Geometry check sheet. Reference: the model listing, model coordinates, mm. A direction names the side the tool comes from. Coordinates: 2 decimals unless noted, no trailing zeros. Loops run counter-clockwise (first coordinate to the right, second up) from the corner with the lowest first, then second, coordinate; pieces in that order, holes last.
from build123d import *

# Parameters (mm, degrees)
F0_W     = 65
F0_H     = 80
F1_DEPTH = 12
F2_T     = 2
F3_W     = 67
F3_H     = 14
F4_DEPTH = 3
F5_W     = 33
F5_H     = 7
F5_W_2   = 39
F5_H_2   = 33
F6_DEPTH = 2


with BuildPart() as f1:
    # F0 (on Front) → F1 (new body)
    with BuildSketch(Plane.XZ):
        with Locations((32.5, 40)):
            Rectangle(F0_W, F0_H)
    extrude(amount=-F1_DEPTH)

    # F2
    f2_openings = [f1.faces().sort_by_distance(p)[0] for p in [
        (32.5, 6, 80),
    ]]
    offset(amount=F2_T, openings=f2_openings, kind=Kind.INTERSECTION)

    # F3 (on face) → F4 (cut)
    with BuildSketch(Plane.XY.offset(80)):
        with Locations((32.5, 6)):
            Rectangle(F3_W, F3_H)
    extrude(amount=-F4_DEPTH, mode=Mode.SUBTRACT)

    # F5 (on face) → F6 (cut, through all)
    with BuildSketch(Plane.XZ.offset(2)):
        with Locations((32.5, 12.5)):
            Rectangle(F5_W, F5_H)
        with Locations((32.5, 56.5)):
            Rectangle(F5_W_2, F5_H_2)
    extrude(amount=-F6_DEPTH, mode=Mode.SUBTRACT)


solid = f1.part
1) Section check A-A on x = 30. Record the cut outline in (y, z).
Data:
outline: (-2, -2) - (14, -2) - (14, 80) - (13, 80) - (13, 77) - (12, 77) - (12, 0) - (0, 0) - (0, 9) - (-2, 9) - close; (-2, 16) - (0, 16) - (0, 40) - (-2, 40) - close; (-2, 73) - (0, 73) - (0, 77) - (-1, 77) - (-1, 80) - (-2, 80) - close
2) Mould release check, pull along X, two halves, no side actions. Record for faces 1 (the flat face through (66, 6, 79)), 2 (the flat face through (32, -2, 39.6)), 3 (the flat face through (-2, 6, 38)): +X half, -X half, draft (parallel to the pull), parting line (faces both ways), or undercut.
Data:
face 1: undercut
face 2: draft
face 3: -X half
3) Section check C-C on y = 10. Record the cut outline in (x, z).
Data:
outline: (-2, -2) - (67, -2) - (67, 80) - (66, 80) - (66, 77) - (65, 77) - (65, 0) - (0, 0) - (0, 77) - (-1, 77) - (-1, 80) - (-2, 80) - close
4) Material ranges on probe 1 along Y at (x, z) = (36, 22.5); probe 2 along X at (y, z) = (2.5, 39); probe 3 along Z at (x, y) = (33.5, 6), recorded low to high.
Data:
probe 1: y = -2 to 0, 12 to 14
probe 2: x = -2 to 0, 65 to 67
probe 3: z = -2 to 0
5) Section check B-B on z = 12. Record the cut outline in (x, y).
Data:
outline: (-2, -2) - (16, -2) - (16, 0) - (0, 0) - (0, 12) - (65, 12) - (65, 0) - (49, 0) - (49, -2) - (67, -2) - (67, 14) - (-2, 14) - close
6) Access from +Z, -Z, +X, -X, +Y, -Y to the whole of each face (thin tool, end or side, straight path). Record for faces 4 (the flat face through (67, 6, 38)), 5 (the flat face through (32, 13, 79)), 6 (the flat face through (16, -1, 12)).
Data:
face 4: +Z, -Z, +X, +Y, -Y
face 5: +Z
face 6: -Y
7) Depth check by flat-ended pin: pin 1 (6 mm diameter, centred on x = 48.5, y = 3.5, fed in from +Z). Enter the tip coordinate at first touch or a pass-through.
Data:
pin 1: stops at z = 0
